Can you work these out from the model? Positions are in its coordinate system, mm. A direction names the side the tool comes from. Round coordinates to 2 decimals unless told otherwise and drop trailing zeros. Loops run counter-clockwise (first coordinate to the right, second up) from the corner with the lowest first, then second, coordinate; pieces in that order, holes last. Notation, with made-up numbers: M -28.75,18.25 L 27.25,18.25 A15 cw 27.25,32.25 Z; hole C 78,22.5 d10. An arc over 180 degrees is marked long. Answer as CSV lines item,"result".
from build123d import *

# Parameters (mm, degrees)
SKETCH_1_W          = 2.5
SKETCH_1_H          = 103
SKETCH_1_W_2        = 2
SKETCH_1_H_2        = 95
EXTRUDE_1_DEPTH     = 63
SKETCH_5_W          = 50
SKETCH_5_H          = 2
EXTRUDE_2_DEPTH     = 11
EXTRUDE_3_DEPTH     = 3
CUT_EXTRUDE_1_DEPTH = 4.5
SKETCH_11_W         = 8.5
SKETCH_11_H         = 11.5
CUT_EXTRUDE_2_DEPTH = 4.5
SKETCH_12_W         = 26
SKETCH_12_H         = 28
SKETCH_12_W_2       = 25
SKETCH_12_H_2       = 27
SKETCH_12_W_3       = 8.5
SKETCH_12_H_3       = 11.5
CUT_EXTRUDE_3_DEPTH = 1
SKETCH_13_W         = 30
SKETCH_13_H         = 2
EXTRUDE_4_DEPTH     = 4
EXTRUDE_5_DEPTH     = 3
SKETCH_15_R         = 0.5
EXTRUDE_6_DEPTH     = 16.933321459


with BuildPart() as part:
    # 스케치1 → 보스-돌출1 (new body)
    with BuildSketch(Plane(origin=(0, 0, 0), x_dir=(1, 0, 0), z_dir=(0, 1, 0))):
        with Locations((-1, 0)):
            Rectangle(SKETCH_1_W, SKETCH_1_H)
        with Locations((1.25, 0)):
            Rectangle(SKETCH_1_W_2, SKETCH_1_H_2)
    extrude(amount=EXTRUDE_1_DEPTH)

    # 스케치5 → 보스-돌출2 (add)
    with BuildSketch(Plane.ZY.offset(2.25)):
        with Locations((0, 1)):
            Rectangle(SKETCH_5_W, SKETCH_5_H)
    extrude(amount=EXTRUDE_2_DEPTH)

    # 스케치7 → 보스-돌출3 (add)
    with BuildSketch(Plane(origin=(0, 2, 0), x_dir=(1, 0, 0), z_dir=(0, 1, 0))):
        Polygon((-2.25, 23), (-11.25, 23), (-11.25, -23), (-2.25, -23), (-2.25, -25), (-13.25, -25), (-13.25, 25), (-2.25, 25), align=None)
    extrude(amount=EXTRUDE_3_DEPTH)

    # 스케치10 → 컷-돌출1 (cut)
    with BuildSketch(Plane(origin=(2.25, 0, 0), x_dir=(0, 0, -1), z_dir=(1, 0, 0))):
        with BuildLine():
            Line((-20.78, 15.25), (-20.78, 12.25))
            ThreePointArc((-20.78, 12.25), (-12.34, 3.81), (-3.9, 12.25))
            Line((-3.9, 12.25), (-3.9, 15.25))
            ThreePointArc((-3.9, 15.25), (-12.34, 23.69), (-20.78, 15.25))
        make_face()
        with BuildLine():
            Line((4.72, 15.25), (4.72, 12.25))
            ThreePointArc((4.72, 12.25), (13.16, 3.81), (21.6, 12.25))
            Line((21.6, 12.25), (21.6, 15.25))
            ThreePointArc((21.6, 15.25), (13.16, 23.69), (4.72, 15.25))
        make_face()
    extrude(amount=-CUT_EXTRUDE_1_DEPTH, mode=Mode.SUBTRACT)

    # 스케치11 → 컷-돌출2 (cut)
    with BuildSketch(Plane.ZY.offset(2.25)):
        with Locations((0, 46.05)):
            Rectangle(SKETCH_11_W, SKETCH_11_H)
    extrude(amount=-CUT_EXTRUDE_2_DEPTH, mode=Mode.SUBTRACT)

    # 스케치12 → 컷-돌출3 (cut)
    # profile 1 of 2: a face of its own
    with BuildSketch(Plane.ZY.offset(2.25)):
        with Locations((0, 43.5)):
            Rectangle(SKETCH_12_W, SKETCH_12_H)
        with Locations((0, 43.5)):
            Rectangle(SKETCH_12_W_2, SKETCH_12_H_2, mode=Mode.SUBTRACT)
    # profile 2 of 2: a face of its own
    with BuildSketch(Plane.ZY.offset(2.25)):
        with Locations((0, 43.5)):
            Rectangle(SKETCH_12_W_2, SKETCH_12_H_2)
        with Locations((0, 46.05)):
            Rectangle(SKETCH_12_W_3, SKETCH_12_H_3, mode=Mode.SUBTRACT)
    extrude(amount=-CUT_EXTRUDE_3_DEPTH, mode=Mode.SUBTRACT)

    # 스케치13 → 보스-돌출4 (add)
    with BuildSketch(Plane.ZY.offset(2.25)):
        with Locations((0, 28.5)):
            Rectangle(SKETCH_13_W, SKETCH_13_H)
    extrude(amount=EXTRUDE_4_DEPTH)

    # 스케치14 → 보스-돌출5 (add)
    with BuildSketch(Plane(origin=(0, 29.5, 0), x_dir=(1, 0, 0), z_dir=(0, 1, 0))):
        Polygon((-2.25, -13), (-2.25, -15), (-6.25, -15), (-6.25, 15), (-2.25, 15), (-2.25, 13), (-4.25, 13), (-4.25, -13), align=None)
    extrude(amount=EXTRUDE_5_DEPTH)

    # 스케치15 → 보스-돌출6 (add)
    with BuildSketch(Plane.XY.offset(51.5)):
        with Locations(Location((-1, 3.34687428, 0), (0, 0, 180))):
            Circle(SKETCH_15_R)
        with Locations(Location((-1, 17.34687428, 0), (0, 0, 180))):
            Circle(SKETCH_15_R)
        with Locations(Location((-1, 31.34687428, 0), (0, 0, 180))):
            Circle(SKETCH_15_R)
        with Locations(Location((-1, 45.34687428, 0), (0, 0, 180))):
            Circle(SKETCH_15_R)
        with Locations(Location((-1, 59.34687428, 0), (0, 0, 180))):
            Circle(SKETCH_15_R)
    extrude(amount=EXTRUDE_6_DEPTH)


solid = part.part
Item 1: We'd pull the mould along Y, two halves only. Please class faces 5 (the face through (-5, 32.5, 0)), 6 (the face through (-4, 27.5, 0)), 7 (the face through (-4.25, 31, 0)), 8 (the face through (-4, 0, -1)): released by +Y, released by -Y, zero draft, split by the parting line, or undercut.
Output:
face 5,"released by +Y"
face 6,"undercut"
face 7,"zero draft"
face 8,"released by -Y"
Item 2: On a 3-axis mill with a long thin cutter (end or side, diameter ignored), from which of +Z, -Z, +X, -X, +Y, -Y can I reach the whole of each face in a straight line? I mean faces 1 (the face through (0.031, 3.812, -12.974)), 2 (the face through (0.25, 31, -49)), 3 (the face through (-4, 30, -15)), 4 (the face through (-8, 2, 25)). Say none if no direction works.
Output:
face 1,"+X"
face 2,"-Z, +X, +Y, -Y"
face 3,"-Z, -X, +Y"
face 4,"+Z, -X, +Y, -Y"
Item 3: If I drill on line 1 along Z through (x, y) = (-5, 4.5); line 2 along X through (y, z) = (4, -30.5); line 3 along Y through (x, z) = (-7, -14.5), over which ranges is the centre line in solid material (lowest first)? Write a range as from..to.
Output:
line 1,"z = -25..-23, 23..25"
line 2,"x = -2.25..2.25"
line 3,"y = 0..2"
Item 4: If we section it at A-A on x = -7.75: Write out the boundary of the cut face in (y, z), then the cut area to 3 significant figures.
Output:
outline,"M 0,-25 L 5,-25 L 5,-23 L 2,-23 L 2,23 L 5,23 L 5,25 L 0,25 Z"
area,"112 mm2"
Item 5: If we section it at B-B on z = 41: Write out the boundary of the cut face in (x, y), then the cut area to 4 significant figures.
Output:
outline,"M -2.25,0 L 2.25,0 L 2.25,63 L -2.25,63 Z"
area,"283.5 mm2"
Item 6: Will these pins go through, and if not, where does the flat tip stop? pin 1 (3.5 mm diameter, centred on x = -1, y = 14.5, fed in from +Z); pin 2 (3 mm diameter, centred on y = 7, z = -35.5, fed in from -X); pin 3 (4 mm diameter, centred on x = -9.5, y = 3, fed in from +Z).
Output:
pin 1,"stops at z = 51.5"
pin 2,"stops at x = -2.25"
pin 3,"stops at z = 25"
